Design review of the part built by this model. Coordinates are the model's own, in mm. Coordinates: 2 decimals unless noted, no trailing zeros. One line per item, written item: value. Start each with the question number.
1. Add section A-A on z = 3.45. Give the number of separate pieces and of enclosed holes in the cut face, plus the area to 3 significant figures.
2. Insertion check: pin 1 (1.8 mm diameter, centred on x = 226.15, y = -7.7, fed in from +Z); pin 2 (3.5 mm diameter, centred on x = 7.7, y = 0, fed in from +Z); pin 3 (3 mm diameter, centred on y = -6, z = 4, fed in from +X); pin 4 (1.5 mm diameter, centred on y = -2.5, z = 3, fed in from +X). Each pin has a flat end and moves straight along its axis. Give the tip position at first contact, or say it passes through.
3. For probe 1 along Y at (x, z) = (0, 2.3); probe 2 along X at (y, z) = (-6.5, 0.65); probe 3 along X at (y, z) = (7.7, 1.5), list the stretches that pass through material, from the lowest coordinate up.
```python
from build123d import *

# Parameters (mm, degrees)
SKETCH1_R           = 1.5
BOSS_EXTRUDE1_DEPTH = 5.4


with BuildPart() as part:
    # Sketch1 → Boss-Extrude1 (new body)
    with BuildSketch(Plane.XY):
        with BuildLine():
            Line((0, -15), (226.153846154, -15))
            ThreePointArc((226.153846154, -15), (241.153846154, 0), (226.153846154, 15))
            Line((226.153846154, 15), (0, 15))
            ThreePointArc((0, 15), (-15, 0), (0, -15))
        make_face()
        with Locations(Location((0, 7.7, 0), (0, 0, 180))):
            Circle(SKETCH1_R, mode=Mode.SUBTRACT)
        with Locations(Location((7.7, 0, 0), (0, 0, 180))):
            Circle(SKETCH1_R, mode=Mode.SUBTRACT)
        with Locations(Location((0, -7.7, 0), (0, 0, 180))):
            Circle(SKETCH1_R, mode=Mode.SUBTRACT)
        with Locations(Location((-7.7, 0, 0), (0, 0, 180))):
            Circle(SKETCH1_R, mode=Mode.SUBTRACT)
        with Locations(Location((218.453846154, 0, 0), (0, 0, 180))):
            Circle(SKETCH1_R, mode=Mode.SUBTRACT)
        with Locations(Location((226.153846154, -7.7, 0), (0, 0, 180))):
            Circle(SKETCH1_R, mode=Mode.SUBTRACT)
        with Locations(Location((233.853846154, 0, 0), (0, 0, 180))):
            Circle(SKETCH1_R, mode=Mode.SUBTRACT)
        with Locations(Location((226.153846154, 7.7, 0), (0, 0, 180))):
            Circle(SKETCH1_R, mode=Mode.SUBTRACT)
    extrude(amount=BOSS_EXTRUDE1_DEPTH)


solid = part.part
```
Worked answers:
1. separate pieces: 1
1. enclosed holes: 8
1. area: 7,430 mm²
2. pin 1: passes through
2. pin 2: stops at z = 5.4
2. pin 3: stops at x = 240.46
2. pin 4: stops at x = 241.05
3. probe 1: y = -15 to -9.2, -6.2 to 6.2, 9.2 to 15
3. probe 2: x = -13.52 to -0.9, 0.9 to 225.25, 227.05 to 239.67
3. probe 3: x = -12.87 to -1.5, 1.5 to 224.65, 227.65 to 239.03
